Source: CAD feature listing. Evaluate the final solid. Frame: model axes, mm. A direction names the side the tool comes from. Give positions to 0.01 mm unless a question says otherwise; leave off trailing zeros. Write each loop counter-clockwise with the first axis right and the second up, starting at its lowest first coordinate (ties: lowest second). Pieces come first, ordered by that corner, then holes. Notation, with made-up numbers: (41.5, 56.5) -> (97.5, 56.5) arc R12 ccw to (97.5, 70.5) -> close; hole circle Ø7 at (35.25, -7.75). An arc over 180 degrees is marked (long way). Answer as a JSON object with one key per item and string values. Group by question number.
Item 1: Section query D-D on y = 1. Return the cut outline in (x, z), plus the area to 3 significant figures.
Item 2: Ray query, probe 1 along X at (y, z) = (-4.75, -1.35); probe 2 along X at (y, z) = (-0.5, 1.1); probe 3 along Y at (x, z) = (2.25, 1.3). Return the intervals inside material, ascending. Write a range as from..to.
Item 3: First-contact query: pin 1 Ø1 at (x, z) = (9.5, 0) entering from +Y; pin 2 Ø2.5 at (x, y) = (5.5, -3.5) entering from +Z (3 decimals); pin 3 Ø0.5 at (y, z) = (-0.5, -1.5) entering from -X; pin 4 Ø0.5 at (y, z) = (-0.5, 1) entering from +X. Flat tips, straight axial feed; report the tip coordinate or a pass-through.
Item 4: Section query A-A on y = -4.25. Return the cut outline in (x, z) (3 decimals).
Item 5: Section query B-B on z = 0. Return the cut outline in (x, y).
Item 6: Section query C-C on x = 9.5. Return the cut outline in (y, z) (1 decimal), plus the area to 3 significant figures.
Item 7: Access query for faces 1 (the face through (-0.715, 1.588, 1.375)), 2 (the face through (6.2, -2.3, -1.045)), 3 (the face through (6.3, -2.5, 1.3)), 4 (the face through (6.2, -2.3, 1.495)). Directions: +Z, -Z, +X, -X, +Y, -Y. A direction counts if a zero-diameter tool reaches every point of the face in a straight line with its end or side. Return the directions, or none.
from build123d import *

# Parameters (mm, degrees)
SKETCH2_W = 0.4
SKETCH2_H = 0.45


with BuildPart() as part:
    # Sketch1 → Revolve1 (revolve)
    with BuildSketch(Plane.XY):
        with BuildLine():
            Line((0, 0), (-1.5, 0))
            ThreePointArc((-1.5, 0), (-1.596592583, 0.074118095), (-1.55, 0.18660254))
            Line((-1.55, 0.18660254), (-1.55, 2.95))
            ThreePointArc((-1.55, 2.95), (-1.096015511, 4.046015511), (0, 4.5))
            Line((0, 4.5), (0, 0))
        make_face()
    revolve(axis=Axis((0, 4.5, 0), (0, -1, 0)))

    # Sweep1: sweep along a path in Sketch4
    with BuildLine(Plane.XY) as sweep1_path:
        Line((0, 0), (0, -0.8))
        ThreePointArc((0, -0.8), (0.092564776, -1.055897602), (0.327417914, -1.193359684))
        Line((0.327417914, -1.193359684), (12.112582086, -3.367938908))
        ThreePointArc((12.112582086, -3.367938908), (12.347435224, -3.505400989), (12.44, -3.761298592))
        Line((12.44, -3.761298592), (12.44, -5.361298592))
    # Sketch2 → Sweep1 (sweep)
    with BuildSketch(Plane.XZ):
        with Locations((0, 1.27)):
            Rectangle(SKETCH2_W, SKETCH2_H)
        with Locations((0, -1.27)):
            Rectangle(SKETCH2_W, SKETCH2_H)
    sweep(path=sweep1_path.line)


solid = part.part
Worked answers:
{
 "1": {"outline": "circle Ø3.1 at (0, 0)", "area": "7.55 mm^2"},
 "2": {"probe 1": "12.24..12.64", "probe 2": "-0.2..0.2", "probe 3": "-1.75..-1.34"},
 "3": {"pin 1": "through", "pin 2": "z = 1.495", "pin 3": "x = -0.2", "pin 4": "x = 0.2"},
 "4": {"outline": "(12.24, -1.495) -> (12.64, -1.495) -> (12.64, -1.045) -> (12.24, -1.045) -> close; (12.24, 1.045) -> (12.64, 1.045) -> (12.64, 1.495) -> (12.24, 1.495) -> close"},
 "5": {"outline": "(-1.55, 0.19) arc R0.1 ccw to (-1.5, 0) -> (1.5, 0) arc R0.1 ccw to (1.55, 0.19) -> (1.55, 2.95) arc R1.55 ccw to (-1.55, 2.95) -> close"},
 "6": {"outline": "(-3.1, -1.5) -> (-2.7, -1.5) -> (-2.7, -1) -> (-3.1, -1) -> close; (-3.1, 1) -> (-2.7, 1) -> (-2.7, 1.5) -> (-3.1, 1.5) -> close", "area": "0.366 mm^2"},
 "7": {"face 1": "+Y", "face 2": "+X, -X, -Y", "face 3": "+Z, -Z, -X, -Y", "face 4": "+Z, +X, -X, -Y"}
}
